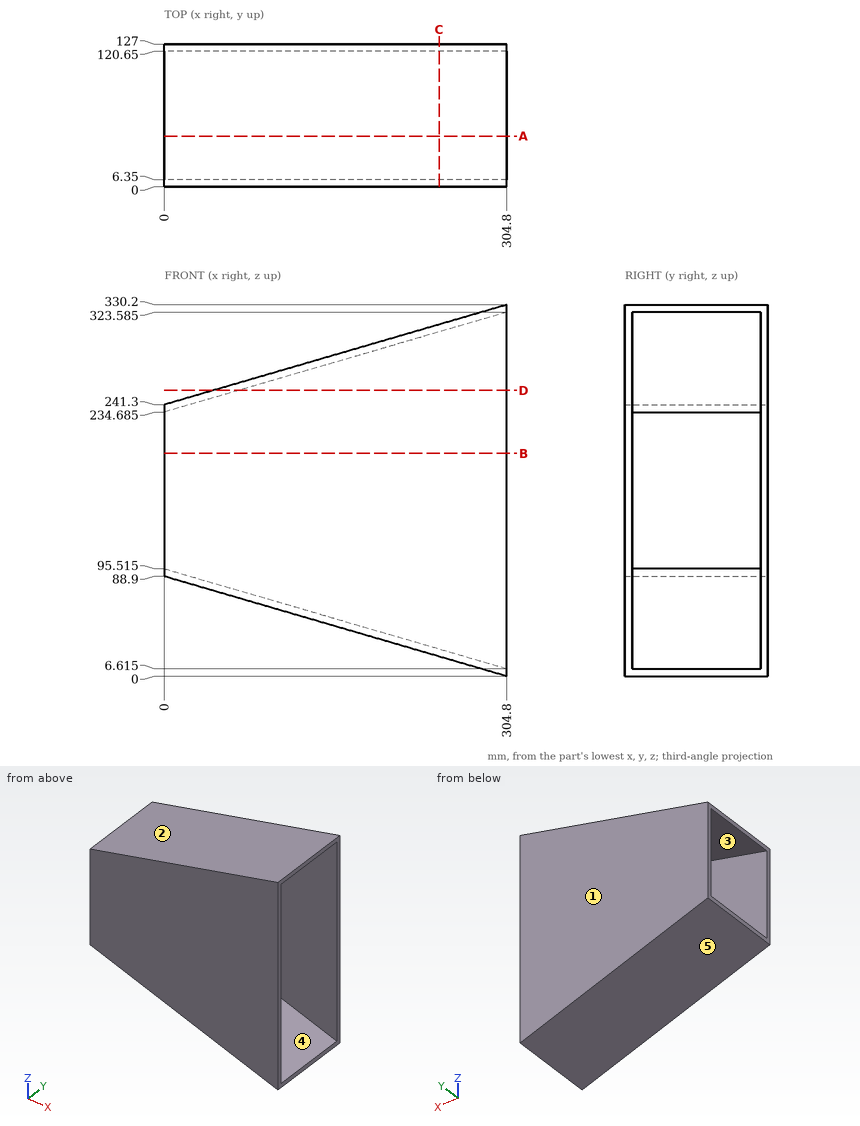
Here's the drawing with two shaded views (mm, measured from the low corner). I have some questions. A direction names the side the tool comes from. Coordinates: 2 decimals unless noted, no trailing zeros. Order: outer loops, then holes, each group sorted by start corner. A loop starts at its lowest first (then second) coordinate and runs counter-clockwise, first axis right, second up. Notation, with made-up numbers: M 87.25,73.5 L 106.25,73.5 A16 cw 106.25,99.5 Z; hole C 64.25,-37.5 d5. An arc over 180 degrees is marked long. Write item = value, one per line.
(1) Suppose I cut it at A-A on y = 45. Please give me the cut outline in (x, z) (1 decimal).
Results are:
outline = M 0,88.9 L 304.8,0 L 304.8,6.6 L 0,95.5 Z; M 0,234.7 L 304.8,323.6 L 304.8,330.2 L 0,241.3 Z
(2) Suppose I cut it at D-D on z = 254. Please give me the cut outline in (x, y).
Results are:
outline = M 43.54,0 L 304.8,0 L 304.8,6.35 L 66.22,6.35 L 66.22,120.65 L 304.8,120.65 L 304.8,127 L 43.54,127 Z
(3) For pin 1 Ø8 at (x, y) = (231, 37) entering from -Z, with a flat end and sliding along its axis, tell me the tip position at first contact or that it passes through.
Results are:
pin_1 = 20.36
(4) I need wall thicknesses on line 1 along Y through (x, z) = (63, 228); line 2 along Z through (x, y) = (191.5, 42.5) (1 decimal); line 3 along Z through (x, y) = (263.5, 117) (1 decimal). Which ranges of each line are inside material? Lowest first, please. Write a range as [from, to].
Results are:
line_1 = [0, 6.35], [120.65, 127]
line_2 = [33, 39.7], [290.5, 297.2]
line_3 = [12, 18.7], [311.5, 318.2]
(5) Suppose I cut it at C-C on x = 244.5. Please give me the cut outline in (y, z), plus the area to 3 significant figures.
Results are:
outline = M 0,17.59 L 127,17.59 L 127,312.61 L 0,312.61 Z; hole M 6.35,24.2 L 120.65,24.2 L 120.65,306 L 6.35,306 Z
area = 5,260 mm2
(6) Suppose I cut it at B-B on z = 198. Please give me the cut outline in (x, y), plus the area to 3 significant figures.
Results are:
outline = M 0,0 L 304.8,0 L 304.8,6.35 L 0,6.35 Z; M 0,120.65 L 304.8,120.65 L 304.8,127 L 0,127 Z
area = 3,870 mm2
(7) For the marked faces 4 and 5, which set-ups out of +Z, -Z, +X, -X, +Y, -Y let a thin tool reach every point of the face, with its end or its side?
Results are:
face_4 = +X
face_5 = -Z, -X, +Y, -Y
(8) If we mould it in two halves opening along Y, with no side actions, what happens to the marked faces 1, 2 and 3? For each: pulls with the +Y half, pulls with the -Y half, needs draft (parallel to the pull), parting line crosses it, or undercut.
Results are:
face_1 = pulls with the +Y half
face_2 = needs draft
face_3 = undercut
